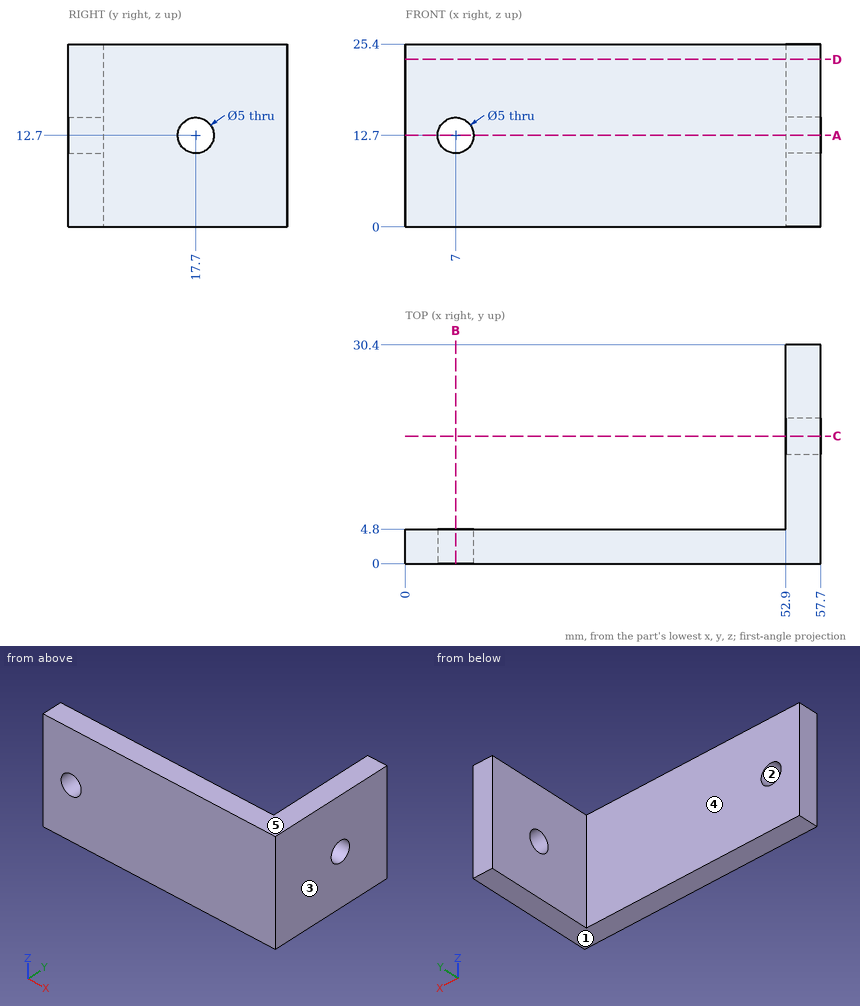
Check sheet for the drawn part. Datum: minimum x, y, z corner. Units: mm. A direction names the side the tool comes from. Give positions to 0.01 mm unless a question says otherwise; leave off trailing zeros. Write each loop counter-clockwise with the first axis right and the second up, starting at its lowest first coordinate (ties: lowest second). Pieces come first, ordered by that corner, then holes.
(1) Material ranges on line 1 (Z direction, x = 56.55, y = 17.7); line 2 (Y direction, x = 44, z = 12.75); line 3 (X direction, y = 25.5, z = 23.5), recorded low to high.
(2) Gauge pin test, flat ends, axial feed: pin 1 (4 mm diameter, centred on y = 20, z = 7, fed in from -X); pin 2 (6 mm diameter, centred on x = 16.5, y = 10, fed in from +Z); pin 3 (12.5 mm diameter, centred on x = 17, z = 11, fed in from +Y). Record the tip position at first contact, or that the pin passes through.
(3) Cross-section at C-C (y = 17.7). Enter the section's corners in (x, z), plus the area to 3 significant figures.
(4) Access from +Z, -Z, +X, -X, +Y, -Y to the whole of each face (thin tool, end or side, straight path). Record for the marked faces 4 and 5.
(5) Cross-section at B-B (x = 7). Enter the section's corners in (y, z), plus the area to 3 significant figures.
(6) Mould release check, pull along Z, two halves, no side actions. Record for the marked faces 1, 2 and 3: +Z half, -Z half, draft (parallel to the pull), parting line (faces both ways), or undercut.
(7) Cross-section at A-A (z = 12.7). Enter the section's corners in (x, y).
(8) Cross-section at D-D (z = 23.25). Enter the section's corners in (x, y).
Worked out:
1. line 1: z = 0 to 10.2, 15.2 to 25.4
1. line 2: y = 0 to 4.8
1. line 3: x = 52.9 to 57.7
2. pin 1: stops at x = 52.9
2. pin 2: passes through
2. pin 3: stops at y = 4.8
3. outline: (52.9, 0) - (57.7, 0) - (57.7, 10.2) - (52.9, 10.2) - close; (52.9, 15.2) - (57.7, 15.2) - (57.7, 25.4) - (52.9, 25.4) - close
3. area: 97.9 mm2
4. face 4: +Z, -Z, -X, +Y
4. face 5: +Z, +X, -X, +Y, -Y
5. outline: (0, 0) - (4.8, 0) - (4.8, 10.2) - (0, 10.2) - close; (0, 15.2) - (4.8, 15.2) - (4.8, 25.4) - (0, 25.4) - close
5. area: 97.9 mm2
6. face 1: -Z half
6. face 2: undercut
6. face 3: draft
7. outline: (0, 0) - (4.5, 0) - (4.5, 4.8) - (0, 4.8) - close; (9.5, 0) - (57.7, 0) - (57.7, 15.2) - (52.9, 15.2) - (52.9, 4.8) - (9.5, 4.8) - close; (52.9, 20.2) - (57.7, 20.2) - (57.7, 30.4) - (52.9, 30.4) - close
8. outline: (0, 0) - (57.7, 0) - (57.7, 30.4) - (52.9, 30.4) - (52.9, 4.8) - (0, 4.8) - close
